Source: CAD feature listing. Evaluate the final solid. Frame: model axes, mm. Face numbers are marked on the shaded views. Give positions to 0.01 mm unless a question says otherwise; leave off trailing zeros. Write each loop counter-clockwise with the first axis right and the second up, starting at its lowest first coordinate (ties: lowest second). Pieces come first, ordered by that corner, then holes.
```python
from build123d import *

# Parameters (mm, degrees)
SKETCH1_R                     = 20
SKETCH1_R_2                   = 17.75
BOSS_EXTRUDE1_DEPTH           = 9
SKETCH2_R                     = 17.75
SKETCH2_R_2                   = 15.375
BOSS_EXTRUDE3_DEPTH           = 4.215
SKETCH4_R                     = 2.8
M3_TAPPING_INSERT_HOLES_DEPTH = 7
EXTRUDE_THIN2_START           = -9
EXTRUDE_THIN2_DEPTH           = 9
THUMB_KNUCKLE_HOLE_START      = -4.5875
SKETCH7_R                     = 15.25
THUMB_KNUCKLE_HOLE_DEPTH      = 106.441707798
SKETCH8_R                     = 1
SKETCH8_R_2                   = 1.6
THUMB_THROUGH_HOLE_S_DEPTH    = 111.029207798
SKETCH9_R                     = 1.1
CENTER_SCREW_THROUGH_DEPTH    = 111.029207798


with BuildPart() as part:
    # Sketch1 → Boss-Extrude1 (new body)
    # profile 1 of 3: a face of its own
    with BuildSketch(Plane(origin=(0, 0, 0), x_dir=(1, 0, 0), z_dir=(0, 1, 0))):
        with BuildLine():
            ThreePointArc((46.554987721, 6.075149623), (47.262334812, 3.074105201), (47.5, 0))
            ThreePointArc((47.5, 0), (9.667891023, -9.056262443), (39.298411056, 16.149225881))
            ThreePointArc((39.298411056, 16.149225881), (0, 28.975470321), (-39.298411056, 16.149225881))
            ThreePointArc((-39.298411056, 16.149225881), (-18.443737557, 17.832108977), (-7.5, 0))
            ThreePointArc((-7.5, 0), (-30.574105201, -19.762334812), (-46.554987721, 6.075149623))
            ThreePointArc((-46.554987721, 6.075149623), (-51.83640533, -24.60085732), (-48.549912051, -55.554205053))
            ThreePointArc((-48.549912051, -55.554205053), (0, -93.502323139), (48.549912051, -55.554205053))
            ThreePointArc((48.549912051, -55.554205053), (51.83640533, -24.60085732), (46.554987721, 6.075149623))
        make_face()
    # profile 2 of 3: a face of its own
    with BuildSketch(Plane(origin=(0, 0, 0), x_dir=(1, 0, 0), z_dir=(0, 1, 0))):
        with Locations((-27.5, 0)):
            Circle(SKETCH1_R)
        with Locations(Location((-27.5, 0, 0), (0, 0, 270))):
            Circle(SKETCH1_R_2, mode=Mode.SUBTRACT)
    # profile 3 of 3: a face of its own
    with BuildSketch(Plane(origin=(0, 0, 0), x_dir=(1, 0, 0), z_dir=(0, 1, 0))):
        with Locations((27.5, 0)):
            Circle(SKETCH1_R)
        with Locations(Location((27.5, 0, 0), (0, 0, 270))):
            Circle(SKETCH1_R_2, mode=Mode.SUBTRACT)
    extrude(amount=BOSS_EXTRUDE1_DEPTH)

    # Sketch2 → Boss-Extrude3 (add)
    # profile 1 of 2: a face of its own
    with BuildSketch(Plane(origin=(0, 0, 0), x_dir=(1, 0, 0), z_dir=(0, 1, 0))):
        with Locations(Location((-27.5, 0, 0), (0, 0, 270))):
            Circle(SKETCH2_R)
        with Locations(Location((-27.5, 0, 0), (0, 0, 270))):
            Circle(SKETCH2_R_2, mode=Mode.SUBTRACT)
    # profile 2 of 2: a face of its own
    with BuildSketch(Plane(origin=(0, 0, 0), x_dir=(1, 0, 0), z_dir=(0, 1, 0))):
        with Locations(Location((27.5, 0, 0), (0, 0, 270))):
            Circle(SKETCH2_R)
        with Locations(Location((27.5, 0, 0), (0, 0, 270))):
            Circle(SKETCH2_R_2, mode=Mode.SUBTRACT)
    extrude(amount=BOSS_EXTRUDE3_DEPTH)

    # Sketch4 → M3_Tapping_Insert_Holes (cut)
    with BuildSketch(Plane(origin=(0, 9, 0), x_dir=(1, 0, 0), z_dir=(0, 1, 0))):
        with Locations(Location((-8, 21.01, 0), (0, 0, 270))):
            Circle(SKETCH4_R)
        with Locations(Location((0, -18, 0), (0, 0, 270))):
            Circle(SKETCH4_R)
        with Locations(Location((-40, -22.9303, 0), (0, 0, 270))):
            Circle(SKETCH4_R)
        with Locations(Location((-37.75, -31.5038, 0), (0, 0, 270))):
            Circle(SKETCH4_R)
        with Locations(Location((-40, -40.255, 0), (0, 0, 270))):
            Circle(SKETCH4_R)
        with Locations(Location((-40.5, -52.3285, 0), (0, 0, 270))):
            Circle(SKETCH4_R)
        with Locations(Location((-13, -83, 0), (0, 0, 270))):
            Circle(SKETCH4_R)
        with Locations(Location((40, -40.255, 0), (0, 0, 90))):
            Circle(SKETCH4_R)
        with Locations(Location((37.75, -31.5038, 0), (0, 0, 90))):
            Circle(SKETCH4_R)
        with Locations(Location((40, -22.9303, 0), (0, 0, 90))):
            Circle(SKETCH4_R)
        with Locations(Location((8, 21.01, 0), (0, 0, 90))):
            Circle(SKETCH4_R)
    extrude(amount=-M3_TAPPING_INSERT_HOLES_DEPTH, mode=Mode.SUBTRACT)

    # Sketch5 → Extrude-Thin2 (add)
    with BuildSketch(Plane(origin=(0, 9, 0), x_dir=(1, 0, 0), z_dir=(0, 1, 0)).offset(EXTRUDE_THIN2_START)):
        with BuildLine():
            ThreePointArc((-50.490710842, -56.037216511), (-53.894544169, -27.770971196), (-50.251676697, 0.465463106))
            ThreePointArc((-50.251676697, 0.465463106), (-44.064896745, 13.114076138), (-33.394207534, 22.301026099))
            ThreePointArc((-33.394207534, 22.301026099), (0, 30.975470321), (33.394207534, 22.301026099))
            ThreePointArc((33.394207534, 22.301026099), (44.064896745, 13.114076138), (50.251676697, 0.465463106))
            ThreePointArc((50.251676697, 0.465463106), (53.894544169, -27.770971196), (50.490710842, -56.037216511))
            ThreePointArc((50.490710842, -56.037216511), (0, -95.502323157), (-50.490710842, -56.037216511))
        make_face()
        with BuildLine():
            ThreePointArc((-48.549912048, -55.554205085), (-51.894562065, -27.779432105), (-48.315034049, -0.033951806))
            ThreePointArc((-48.315034049, -0.033951806), (-42.481784381, 11.891883339), (-32.420848839, 20.55386473))
            ThreePointArc((-32.420848839, 20.55386473), (0, 28.975470321), (32.420848839, 20.55386473))
            ThreePointArc((32.420848839, 20.55386473), (42.481784381, 11.891883339), (48.315034049, -0.033951806))
            ThreePointArc((48.315034049, -0.033951806), (51.894562065, -27.779432105), (48.549912048, -55.554205085))
            ThreePointArc((48.549912048, -55.554205085), (0, -93.502323157), (-48.549912048, -55.554205085))
        make_face(mode=Mode.SUBTRACT)
    extrude(amount=EXTRUDE_THIN2_DEPTH)

    # Sketch7 → Thumb_Knuckle_Hole (cut, through all)
    with BuildSketch(Plane(origin=(0, 9, 0), x_dir=(1, 0, 0), z_dir=(0, 1, 0)).offset(THUMB_KNUCKLE_HOLE_START)):
        with Locations(Location((0, -70, 0), (0, 0, 270))):
            Circle(SKETCH7_R)
    extrude(amount=-THUMB_KNUCKLE_HOLE_DEPTH, mode=Mode.SUBTRACT)

    # Sketch8 → Thumb_Through_Hole(s) (cut, through all)
    with BuildSketch(Plane(origin=(0, 9, 0), x_dir=(1, 0, 0), z_dir=(0, 1, 0))):
        with Locations(Location((0, -70, 0), (0, 0, 270))):
            Circle(SKETCH8_R)
        with Locations(Location((0, -61, 0), (0, 0, 270))):
            Circle(SKETCH8_R_2)
        with Locations(Location((0, -79, 0), (0, 0, 270))):
            Circle(SKETCH8_R_2)
    extrude(amount=-THUMB_THROUGH_HOLE_S_DEPTH, mode=Mode.SUBTRACT)

    # Sketch9 → Center_Screw_Through (cut, through all)
    with BuildSketch(Plane(origin=(0, 9, 0), x_dir=(1, 0, 0), z_dir=(0, 1, 0))):
        with Locations(Location((0, -31.5037951, 0), (0, 0, 270))):
            Circle(SKETCH9_R)
    extrude(amount=-CENTER_SCREW_THROUGH_DEPTH, mode=Mode.SUBTRACT)


solid = part.part
```
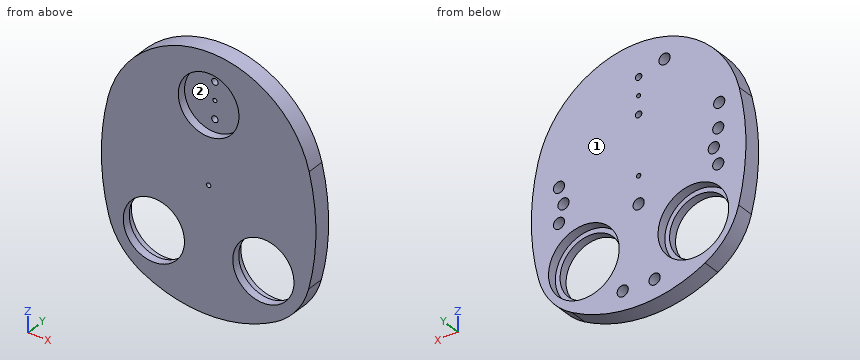
1. Line query: L1, parallel to Z at x = 1, y = 1.75; L2, parallel to Z at x = 37.5, y = 5.75 (3 decimals); L3, parallel to X at y = 4.5, z = -21.01. Output: solid intervals per line, ascending.
2. Mould query, pull axis Z, two halves, no side actions, for the marked faces 1 and 2. Classes: +Z half, -Z half, draft (parallel to the pull), parting line (faces both ways), or undercut.
3. Contact query for flat-ended pins moving along their axis: P1, Ø1.7, axis at x = -41, z = 52.5, coming from the +Y side; P2, Ø3, axis at y = 5.5, z = -1.5, coming from the -X side; P3, Ø5, axis at y = 7, z = -9, coming from the +X side. Output: stop coordinate, or through.
4. Cut plane A-A, the plane y = 6.75. State how many separate pieces and enclosed holes the cut face has, then the cut area to 3 significant figures.
5. Cut plane B-B, the plane x = 13.5. Return the cut outline in (y, z) (1 decimal).
6. Cut plane D-D, the plane z = 61. Return the cut outline in (x, y), then the cut area to 3 significant figures.
7. Cut plane C-C, the plane z = 5. Return the cut outline in (x, y) (3 decimals), then the cut area to 3 significant figures.
Response values:
1. L1: z = -30.97 to 31.05, 31.96 to 54.78, 85.22 to 95.49
1. L2: z = -19.62 to -14.665, 14.665 to 21.669, 24.191 to 28.715, 34.293 to 38.994, 41.516 to 79.54
1. L3: x = -35.53 to -10.8, -5.2 to 5.2, 10.8 to 35.53
2. face 1: draft
2. face 2: undercut
3. P1: stops at y = 2
3. P2: stops at x = -50.37
3. P3: stops at x = 48.09
4. separate pieces: 1
4. enclosed holes: 17
4. area: 8,970 mm2
5. outline: (0, -29.6) - (9, -29.6) - (9, -10.9) - (4.2, -10.9) - (4.2, -6.4) - (0, -6.4) - close; (0, 6.4) - (4.2, 6.4) - (4.2, 10.9) - (9, 10.9) - (9, 93.7) - (0, 93.7) - (0, 77.1) - (4.4, 77.1) - (4.4, 62.9) - (0, 62.9) - close
6. outline: (-48.99, 0) - (-12.31, 0) - (-12.31, 4.41) - (-1.6, 4.41) - (-1.6, 9) - (-48.99, 9) - close; (1.6, 4.41) - (12.31, 4.41) - (12.31, 0) - (48.99, 0) - (48.99, 9) - (1.6, 9) - close
6. area: 758 mm2
7. outline: (-51.52, 0) - (-42.039, 0) - (-42.039, 4.215) - (-44.531, 4.215) - (-44.531, 9) - (-51.52, 9) - close; (-12.961, 0) - (12.961, 0) - (12.961, 4.215) - (10.469, 4.215) - (10.469, 9) - (-10.469, 9) - (-10.469, 4.215) - (-12.961, 4.215) - close; (42.039, 0) - (51.52, 0) - (51.52, 9) - (44.531, 9) - (44.531, 4.215) - (42.039, 4.215) - close
7. area: 356 mm2
